Read the model definition and answer for the solid it produces. Units are mm, in the model's axes. Face numbers are marked on the shaded views. Give positions to 0.01 mm unless a question says otherwise; leave off trailing zeros. Loops run counter-clockwise (first coordinate to the right, second up) from the corner with the lowest first, then second, coordinate; pieces in that order, holes last. Notation, with made-up numbers: (52, 77) -> (102, 77) arc R26 ccw to (102, 93) -> close; hole circle Ø4 at (2.25, -3). An arc over 180 degrees is marked (long way). Write each question's results on one line, items separated by ' | '. Start each with the question number.
Item 1: Section B-B on z = 39.5 is taken. Write down the section's boundary in (x, y), and give its area (3 significant figures).
Item 2: Section C-C on z = 0 is taken. Write down the section's boundary in (x, y), and give its area (4 significant figures).
Item 3: Section A-A on y = 0 is taken. Write down the section's boundary in (x, z), and give its area (3 significant figures).
Item 4: Each of these flat-tipped pins is pushed along its axis until it touches: P1, Ø2, axis at x = -1, z = 29.5, coming from the -Y side; P2, Ø4, axis at y = 12.37, z = -12.37, coming from the +X side; P3, Ø1.5, axis at x = 0.5, y = 19.5, coming from the -Z side. Where does it stop, or does it pass through?
Item 5: Section D-D on y = -29 is taken. Write down the section's boundary in (x, z).
Item 6: Find the intervals of material crossed by line 1 (Y direction, x = 1.6, z = 54.5); line 2 (Y direction, x = -1.65, z = 54.5); line 3 (Y direction, x = -1.95, z = 0), in increasing order.
Item 7: Determine the mould class of the marked faces 1 and 2 for opening direction Z: +Z half, -Z half, draft (parallel to the pull), parting line (faces both ways), or undercut.
```python
from build123d import *

# Parameters (mm, degrees)
CROQUIS1_R                                           = 12.5
SALIENTE_EXTRUIR1_DEPTH                              = 2.5
CROQUIS2_R                                           = 21
CORTAR_EXTRUIR1_DEPTH                                = 1.5
REFRENTADO_PARA_TORNILLO_TAP_N_CON_CABEZ_D           = 3.4
REFRENTADO_PARA_TORNILLO_TAP_N_CON_CABEZ_DEPTH       = 10
REFRENTADO_PARA_TORNILLO_TAP_N_CON_CABEZ_CSINK_D     = 6.72
REFRENTADO_PARA_TORNILLO_TAP_N_CON_CABEZ_CSINK_ANGLE = 90
REFRENTADO_PARA_TORNILLO_TAP_N_CON_CABEZ_TIP         = 1.021463052
TALADRO_DE_MARGEN_PARA_M31_D                         = 3.4
REFRENTADO_PARA_TORNILLO_CON_CABEZA_TRON_D           = 3.4
REFRENTADO_PARA_TORNILLO_CON_CABEZA_TRON_CBORE_D     = 7
REFRENTADO_PARA_TORNILLO_CON_CABEZA_TRON_CBORE_DEPTH = 2.4


with BuildPart() as part:
    # Croquis1 → Saliente-Extruir1 (new, symmetric)
    with BuildSketch(Plane(origin=(0, 0, 0), x_dir=(0, 0, -1), z_dir=(1, 0, 0))):
        with BuildLine():
            Line((-25.870639729, 20), (-60, 20))
            Line((-60, 20), (-60, -20))
            Line((-60, -20), (-25.870639729, -20))
            ThreePointArc((-25.870639729, -20), (32.7, 0), (-25.870639729, 20))
        make_face()
        Circle(CROQUIS1_R, mode=Mode.SUBTRACT)
    extrude(amount=SALIENTE_EXTRUIR1_DEPTH, both=True)

    # Croquis2 → Cortar-Extruir1 (cut)
    with BuildSketch(Plane.ZY.offset(2.5)):
        Circle(CROQUIS2_R)
    extrude(amount=-CORTAR_EXTRUIR1_DEPTH, mode=Mode.SUBTRACT)

    # Refrentado para tornillo tapón con cabeza plana de clavija de M31
    with Locations(Plane(origin=(2.5, 0, 0), x_dir=(0, 0, -1), z_dir=(1, 0, 0))):
        with Locations((12.374368671, 12.374368671), (-12.374368671, -12.374368671), (-12.374368671, 12.374368671), (12.374368671, -12.374368671)):
            CounterSinkHole(REFRENTADO_PARA_TORNILLO_TAP_N_CON_CABEZ_D / 2, REFRENTADO_PARA_TORNILLO_TAP_N_CON_CABEZ_CSINK_D / 2, depth=REFRENTADO_PARA_TORNILLO_TAP_N_CON_CABEZ_DEPTH, counter_sink_angle=REFRENTADO_PARA_TORNILLO_TAP_N_CON_CABEZ_CSINK_ANGLE)
            with Locations((0, 0, -(REFRENTADO_PARA_TORNILLO_TAP_N_CON_CABEZ_DEPTH + REFRENTADO_PARA_TORNILLO_TAP_N_CON_CABEZ_TIP / 2))):  # 118° drill point
                Cone(0, REFRENTADO_PARA_TORNILLO_TAP_N_CON_CABEZ_D / 2, REFRENTADO_PARA_TORNILLO_TAP_N_CON_CABEZ_TIP, mode=Mode.SUBTRACT)

    # Taladro de margen para M31 (through all)
    with Locations(Plane(origin=(2.5, 0, 0), x_dir=(0, 0, -1), z_dir=(1, 0, 0))):
        with Locations((0, 29), (25.11473671, 14.5), (25.11473671, -14.5), (0, -29), (-25.11473671, -14.5), (-25.11473671, 14.5)):
            Hole(TALADRO_DE_MARGEN_PARA_M31_D / 2)

    # Refrentado para tornillo con cabeza troncocónica de M31 (through all)
    with Locations(Plane(origin=(2.5, 0, 0), x_dir=(0, 0, -1), z_dir=(1, 0, 0))):
        with Locations((-39.5, 15), (-54.5, -15), (-54.5, 15), (-39.5, -15)):
            CounterBoreHole(REFRENTADO_PARA_TORNILLO_CON_CABEZA_TRON_D / 2, REFRENTADO_PARA_TORNILLO_CON_CABEZA_TRON_CBORE_D / 2, REFRENTADO_PARA_TORNILLO_CON_CABEZA_TRON_CBORE_DEPTH)


solid = part.part
```
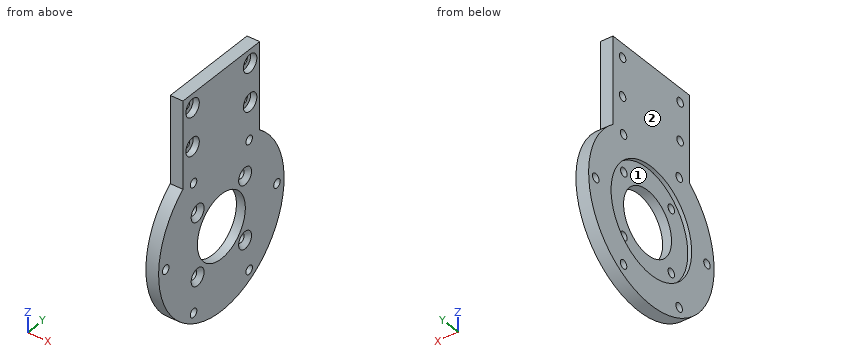
Findings:
1) outline: (-2.5, -20) -> (2.5, -20) -> (2.5, -18.5) -> (0.1, -18.5) -> (0.1, -16.7) -> (-2.5, -16.7) -> close; (-2.5, -13.3) -> (0.1, -13.3) -> (0.1, -11.5) -> (2.5, -11.5) -> (2.5, 11.5) -> (0.1, 11.5) -> (0.1, 13.3) -> (-2.5, 13.3) -> close; (-2.5, 16.7) -> (0.1, 16.7) -> (0.1, 18.5) -> (2.5, 18.5) -> (2.5, 20) -> (-2.5, 20) -> close | area: 149 mm2
2) outline: (-2.5, -32.7) -> (2.5, -32.7) -> (2.5, -30.7) -> (-2.5, -30.7) -> close; (-2.5, -27.3) -> (2.5, -27.3) -> (2.5, -12.5) -> (-1, -12.5) -> (-1, -21) -> (-2.5, -21) -> close; (-2.5, 21) -> (-1, 21) -> (-1, 12.5) -> (2.5, 12.5) -> (2.5, 27.3) -> (-2.5, 27.3) -> close; (-2.5, 30.7) -> (2.5, 30.7) -> (2.5, 32.7) -> (-2.5, 32.7) -> close | area: 142.5 mm2
3) outline: (-2.5, -32.7) -> (2.5, -32.7) -> (2.5, -12.5) -> (-1, -12.5) -> (-1, -21) -> (-2.5, -21) -> close; (-2.5, 21) -> (-1, 21) -> (-1, 12.5) -> (2.5, 12.5) -> (2.5, 60) -> (-2.5, 60) -> close | area: 313 mm2
4) P1: y = -20 | P2: x = 1.15 | P3: z = -26.79
5) outline: (-2.5, -15.11) -> (2.5, -15.11) -> (2.5, -1.7) -> (-2.5, -1.7) -> close; (-2.5, 1.7) -> (2.5, 1.7) -> (2.5, 15.11) -> (-2.5, 15.11) -> close
6) line 1: -20 to -18.5, -11.5 to 11.5, 18.5 to 20 | line 2: -20 to -16.7, -13.3 to 13.3, 16.7 to 20 | line 3: -32.7 to -30.7, -27.3 to -21, 21 to 27.3, 30.7 to 32.7
7) face 1: undercut | face 2: draft
